from build123d import *

# Parameters (mm, degrees)
ESQUISSE1_W        = 48
ESQUISSE1_H        = 40
BOSS_EXTRU_1_DEPTH = 13
CONG_1_R           = 8
CHANFREIN1_SIZE    = 14
CHANFREIN1_SIZE2   = 10.171595392
CONG_2_R           = 8
CHANFREIN2_SIZE    = 5
CHANFREIN2_SIZE2   = 3.63271264


with BuildPart() as part:
    # Esquisse1 → Boss.-Extru.1 (new body)
    with BuildSketch(Plane.XY):
        with Locations((24, 20)):
            Rectangle(ESQUISSE1_W, ESQUISSE1_H)
    extrude(amount=BOSS_EXTRU_1_DEPTH)

    # Congé1
    cong_1_edges = [part.edges().sort_by_distance(p)[0] for p in [
        (0, 40, 6.5),
        (0, 0, 6.5),
    ]]
    fillet(cong_1_edges, radius=CONG_1_R)

    # Chanfrein1
    chanfrein1_edges = [part.edges().sort_by_distance(p)[0] for p in [
        (48, 40, 6.5),
        (48, 0, 6.5),
    ]]
    chanfrein1_side = [part.faces().sort_by_distance(p)[0] for p in [
        (48, 20, 6.5),
    ]]
    chamfer(chanfrein1_edges, length=CHANFREIN1_SIZE, length2=CHANFREIN1_SIZE2, reference=chanfrein1_side[0])

    # Congé2
    cong_2_edges = [part.edges().sort_by_distance(p)[0] for p in [
        (37.828404608, 0, 6.5),
        (37.828404608, 40, 6.5),
    ]]
    fillet(cong_2_edges, radius=CONG_2_R)

    # Chanfrein2
    chanfrein2_edges = [part.edges().sort_by_distance(p)[0] for p in [
        (20.876100506, 0, 13),
        (0, 20, 13),
        (2.343145751, 37.656854249, 13),
        (2.343145751, 2.343145751, 13),
        (48, 20, 13),
        (44.112168483, 31.351141009, 13),
        (20.876100506, 40, 13),
        (44.112168483, 8.648858991, 13),
        (37.38412501, 0.871947806, 13),
        (37.38412501, 39.128052194, 13),
    ]]
    chanfrein2_side = [part.faces().sort_by_distance(p)[0] for p in [
        (22.630137731, 20, 13),
    ]]
    chamfer(chanfrein2_edges, length=CHANFREIN2_SIZE, length2=CHANFREIN2_SIZE2, reference=chanfrein2_side[0])


solid = part.part
Geometry: final body of the model. Coordinates: model frame, mm. Round coordinates to 2 decimals unless told otherwise and drop trailing zeros. Order: outer loops, then holes, each group sorted by start corner. A loop starts at its lowest first (then second) coordinate and runs counter-clockwise, first axis right, second up. Notation, with made-up numbers: (-9.5, 62) - (25.5, 62) arc R29 cw to (25.5, 91) - close; hole circle Ø11 at (-22.75, 50.5). An arc over 180 degrees is marked (long way). Write each question's results on one line, items separated by ' | '.
Item 1: Section D-D, the plane z = 11.75. Return the cut outline in (x, y).
Completed:
outline: (3.28, 8) arc R4.72 ccw to (8, 3.28) - (33.75, 3.28) arc R4.72 ccw to (37.57, 5.23) - (44.72, 15.07) - (44.72, 24.93) - (37.57, 34.77) arc R4.72 ccw to (33.75, 36.72) - (8, 36.72) arc R4.72 ccw to (3.28, 32) - close
Item 2: Section A-A, the plane z = 2.75. Return the cut outline in (x, y), and give its area (3 significant figures).
Completed:
outline: (0, 8) arc R8 ccw to (8, 0) - (33.75, 0) arc R8 ccw to (40.22, 3.3) - (48, 14) - (48, 26) - (40.22, 36.7) arc R8 ccw to (33.75, 40) - (8, 40) arc R8 ccw to (0, 32) - close | area: 1,750 mm^2
Item 3: Section C-C, the plane y = 10. Return the cut outline in (x, z), and give its area (3 significant figures).
Completed:
outline: (0, 0) - (45.09, 0) - (45.09, 9.37) - (38.91, 13) - (5, 13) - (0, 9.37) - close | area: 566 mm^2
Item 4: Section B-B, the plane x = 17.5. Return the cut outline in (y, z).
Completed:
outline: (0, 0) - (40, 0) - (40, 9.37) - (35, 13) - (5, 13) - (0, 9.37) - close
Item 5: First-contact query: pin 1 Ø3 at (y, z) = (27.5, 10) entering from +X. Flat tip, straight axial feed; report the tip coordinate or a pass-through.
Completed:
pin 1: x = 47.9
Item 6: Material intervals for line 1 along Y through (x, z) = (26.5, 11.5); line 2 along Y through (x, z) = (43, 2.25); line 3 along X through (y, z) = (7, 3), sorted ascending. Write a range as [from, to].
Completed:
line 1: [2.94, 37.06] | line 2: [7.12, 32.88] | line 3: [0.06, 42.91]
